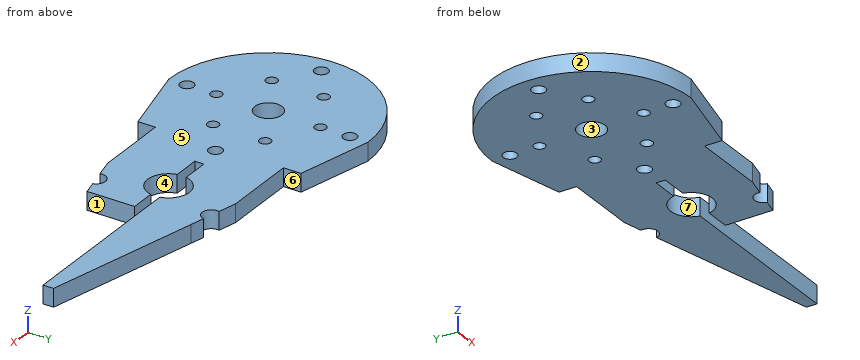
from build123d import *

# Parameters (mm, degrees)
SKETCH_1_R          = 3
SKETCH_1_R_2        = 1.25
SKETCH_1_R_3        = 1.5
EXTRUDE_1_DEPTH     = 4
SKETCH_2_R          = 2
SKETCH_2_W          = 18.21777686
SKETCH_2_H          = 14.090430323
CUT_EXTRUDE_1_DEPTH = 4


with BuildPart() as part:
    # 草图1 → 凸台-拉伸1 (new body)
    with BuildSketch(Plane.XY):
        with BuildLine():
            Line((-15.488984032, 1), (-9.488984032, 1))
            ThreePointArc((-9.488984032, 1), (-4.998995168, 4.6), (-0.509006304, 1))
            Line((-0.509006304, 1), (5.001004832, 1))
            Line((5.001004832, 1), (39.254812875, 1))
            Line((39.254812875, 1), (39.254812875, 3.326018382))
            Line((39.254812875, 3.326018382), (5.001004832, 11.501004832))
            Line((5.001004832, 11.501004832), (-38.998995168, 22.002009663))
            ThreePointArc((-38.998995168, 22.002009663), (-61.001004832, 0), (-38.998995168, -22.002009663))
            Line((-38.998995168, -22.002009663), (5.001004832, -11.501004832))
            Line((5.001004832, -11.501004832), (5.001004832, -1))
            Line((5.001004832, -1), (-0.509006304, -1))
            ThreePointArc((-0.509006304, -1), (-4.998995168, -4.6), (-9.488984032, -1))
            Line((-9.488984032, -1), (-15.488984032, -1))
            Line((-15.488984032, -1), (-15.488984032, 1))
        make_face()
        with Locations((-38.998995168, 0)):
            Circle(SKETCH_1_R, mode=Mode.SUBTRACT)
        with Locations((-38.998995168, -11.5)):
            Circle(SKETCH_1_R_2, mode=Mode.SUBTRACT)
        with Locations((-48.958287312, -5.75)):
            Circle(SKETCH_1_R_2, mode=Mode.SUBTRACT)
        with Locations((-48.958287312, 5.75)):
            Circle(SKETCH_1_R_2, mode=Mode.SUBTRACT)
        with Locations((-38.998995168, 11.5)):
            Circle(SKETCH_1_R_2, mode=Mode.SUBTRACT)
        with Locations((-29.039703025, 5.75)):
            Circle(SKETCH_1_R_2, mode=Mode.SUBTRACT)
        with Locations((-29.039703025, -5.75)):
            Circle(SKETCH_1_R_2, mode=Mode.SUBTRACT)
        with Locations((-38.998995168, -18.002009663)):
            Circle(SKETCH_1_R_3, mode=Mode.SUBTRACT)
        with Locations((-38.998995168, 18.002009663)):
            Circle(SKETCH_1_R_3, mode=Mode.SUBTRACT)
        with Locations((-57.001004832, 0)):
            Circle(SKETCH_1_R_3, mode=Mode.SUBTRACT)
        with Locations((-20.996985505, 0)):
            Circle(SKETCH_1_R_3, mode=Mode.SUBTRACT)
    extrude(amount=EXTRUDE_1_DEPTH)

    # 草图2 → 切除-拉伸1 (cut)
    with BuildSketch(Plane(origin=(0, 0, 0), x_dir=(-1, 0, 0), z_dir=(0, 0, -1))):
        with Locations((0, 12.694540648)):
            Circle(SKETCH_2_R)
        with Locations((0, -12.694540648)):
            Circle(SKETCH_2_R)
        with Locations((13.221008307, 21.185215162)):
            Rectangle(SKETCH_2_W, SKETCH_2_H)
        with Locations((13.221008307, -21.185215162)):
            Rectangle(SKETCH_2_W, SKETCH_2_H)
    extrude(amount=-CUT_EXTRUDE_1_DEPTH, mode=Mode.SUBTRACT)


solid = part.part
Part model, mm, in its own coordinate system. Face numbers are marked on the shaded views. A direction names the side the tool comes from. Give positions to 0.01 mm unless a question says otherwise; leave off trailing zeros. Write each loop counter-clockwise with the first axis right and the second up, starting at its lowest first coordinate (ties: lowest second). Pieces come first, ordered by that corner, then holes.
1) Cut at A-A on y = -5.75. Write the cut outline in (x, z).
Resolved:
outline: (-60.24, 0) - (-50.21, 0) - (-50.21, 4) - (-60.24, 4) - close; (-47.71, 0) - (-30.29, 0) - (-30.29, 4) - (-47.71, 4) - close; (-27.79, 0) - (5, 0) - (5, 4) - (-27.79, 4) - close
2) Pin check, flat tips, straight feed: pin 1 (2.5 mm diameter, centred on x = -39, y = -18, fed in from +Z); pin 2 (1.9 mm diameter, centred on y = -17, z = 2.5, fed in from +X); pin 3 (2 mm diameter, centred on y = -6, z = 1, fed in from +X); pin 4 (0.6 mm diameter, centred on y = 0.5, z = 3, fed in from +X). Stop position of each tip, or through.
Resolved:
pin 1: passes through
pin 2: stops at x = -22.33
pin 3: stops at x = 5
pin 4: stops at x = -15.49
3) Cut at C-C on x = -18.5. Write the cut outline in (y, z), then the cut area to 3 significant figures.
Resolved:
outline: (-14.14, 0) - (14.14, 0) - (14.14, 4) - (-14.14, 4) - close
area: 113 mm2
4) Cut at D-D on x = -51.5. Write the cut outline in (y, z).
Resolved:
outline: (-18.11, 0) - (18.11, 0) - (18.11, 4) - (-18.11, 4) - close
5) Probe L1, parallel to Y at x = -12.5, z = 2.1; L2, parallel to X at y = -2, z = 1.9; L3, parallel to Y at x = -29, z = 2.25. List the from-to ranges inside material, lowest first.
Resolved:
L1: y = -14.14 to -1, 1 to 14.14
L2: x = -60.91 to -41.24, -36.76 to -9.14, -0.86 to 5
L3: y = -19.62 to -7, -4.5 to 4.5, 7 to 19.62
6) Cut at B-B on z = 1.35. State how many separate pieces and enclosed holes the cut face has, then the cut area to 3 significant figures.
Resolved:
separate pieces: 1
enclosed holes: 11
area: 2,200 mm2
7) Which spindle directions (+Z, -Z, +X, -X, +Y, -Y) get a long thin tool onto all of the face, cutting with end or side? Do the marked faces 5, 6 and 7. Say none if no direction does.
Resolved:
face 5: +Z, +X, -X, +Y, -Y
face 6: +Z, -Z, +X, +Y
face 7: +Z, -Z
8) Two-plate mould, pull along X, no slides. Class the marked faces 1, 2, 3 and 4: released by +X, released by -X, zero draft, split by the parting line, or undercut.
Resolved:
face 1: released by +X
face 2: released by -X
face 3: undercut
face 4: undercut
